from build123d import *

# Parameters (mm, degrees)
CROQUIS1_W              = 100
CROQUIS1_H              = 100
SALIENTE_EXTRUIR1_DEPTH = 10
CROQUIS2_R              = 1.5
CORTAR_EXTRUIR1_DEPTH   = 30
CROQUIS3_W              = 7.071067812
CROQUIS3_H              = 7.071067812
CORTAR_EXTRUIR2_DEPTH   = 8
VACIADO1_START          = -48
VACIADO1_OUTLINE_W      = 8
VACIADO1_OUTLINE_H      = 81.857864376
VACIADO1_DEPTH          = 96
VACIADO1_START_2        = -40.928932188
VACIADO1_2_OUTLINE_W    = 8
VACIADO1_2_OUTLINE_H    = 7.071067812
VACIADO1_2_DEPTH        = 81.857864376


# Read off the part's stored shape, not the designer's step: Vaciado1
with BuildPart() as part:
    # Croquis1 → Saliente-Extruir1 (new body)
    with BuildSketch(Plane(origin=(0, 0, 0), x_dir=(1, 0, 0), z_dir=(0, 1, 0))):
        Rectangle(CROQUIS1_W, CROQUIS1_H)
    extrude(amount=SALIENTE_EXTRUIR1_DEPTH)

    # Croquis2 → Cortar-Extruir1 (cut)
    with BuildSketch(Plane(origin=(0, 10, 0), x_dir=(1, 0, 0), z_dir=(0, 1, 0))):
        with Locations(Location((-46.464466094, -46.464466094, 0), (0, 0, 270))):
            Circle(CROQUIS2_R)
        with Locations(Location((-46.464466094, 46.464466094, 0), (0, 0, 270))):
            Circle(CROQUIS2_R)
        with Locations(Location((46.464466094, 46.464466094, 0), (0, 0, 270))):
            Circle(CROQUIS2_R)
        with Locations(Location((46.464466094, -46.464466094, 0), (0, 0, 270))):
            Circle(CROQUIS2_R)
    extrude(amount=-CORTAR_EXTRUIR1_DEPTH, mode=Mode.SUBTRACT)

    # Croquis3 → Cortar-Extruir2 (cut)
    with BuildSketch(Plane(origin=(0, 10, 0), x_dir=(1, 0, 0), z_dir=(0, 1, 0))):
        with Locations((-46.464466094, -46.464466094)):
            Rectangle(CROQUIS3_W, CROQUIS3_H)
        with Locations((-46.464466094, 46.464466094)):
            Rectangle(CROQUIS3_W, CROQUIS3_H)
        with Locations((46.464466094, 46.464466094)):
            Rectangle(CROQUIS3_W, CROQUIS3_H)
        with Locations((46.464466094, -46.464466094)):
            Rectangle(CROQUIS3_W, CROQUIS3_H)
    extrude(amount=-CORTAR_EXTRUIR2_DEPTH, mode=Mode.SUBTRACT)

    # Vaciado1 outline → Vaciado1 (cut)
    with BuildSketch(Plane.YZ.offset(VACIADO1_START)):
        with Locations((4, 0)):
            Rectangle(VACIADO1_OUTLINE_W, VACIADO1_OUTLINE_H)
    extrude(amount=VACIADO1_DEPTH, mode=Mode.SUBTRACT)

    # Vaciado1 2 outline → Vaciado1 2 (cut)
    with BuildSketch(Plane.YZ.offset(VACIADO1_START_2)):
        with Locations((4, -44.464466094)):
            Rectangle(VACIADO1_2_OUTLINE_W, VACIADO1_2_OUTLINE_H)
        with Locations((4, 44.464466094)):
            Rectangle(VACIADO1_2_OUTLINE_W, VACIADO1_2_OUTLINE_H)
    extrude(amount=VACIADO1_2_DEPTH, mode=Mode.SUBTRACT)


solid = part.part
Part model, mm, in its own coordinate system. A direction names the side the tool comes from. Round coordinates to 2 decimals unless told otherwise and drop trailing zeros. Write each loop counter-clockwise with the first axis right and the second up, starting at its lowest first coordinate (ties: lowest second). Pieces come first, ordered by that corner, then holes. Notation, with made-up numbers: M 85.25,37.25 L 128.25,37.25 A37 ccw 128.25,75.25 Z; hole C 73.25,11.5 d11. An arc over 180 degrees is marked long. Return JSON: item names as keys, results as strings. Group by question number.
(1) Drill centre lines: probe 1 along Z at (x, y) = (41.5, 5.75); probe 2 along X at (y, z) = (7, 11). Where is each one in solid material? Low to high.
(2) Saw through at C-C on z = 37.5. Write the cut outline in (x, y), then the cut area to 3 significant figures.
(3) Saw through at A-A on y = 4. Write the cut outline in (x, z), then the cut area to 3 significant figures.
(4) Saw through at B-B on x = 37. Write the cut outline in (y, z), then the cut area to 3 significant figures.
(5) Pin check, flat tips, straight feed: pin 1 Ø6 at (x, z) = (17, -20) entering from -Y; pin 2 Ø3.5 at (y, z) = (6, 46) entering from +X; pin 3 Ø5.5 at (x, y) = (46.5, 5.5) entering from -Z; pin 4 Ø1.8 at (x, z) = (46.46, 46.46) entering from -Y. Stop position of each tip, or through.
(6) Which spindle directions (+Z, -Z, +X, -X, +Y, -Y) get a long thin tool onto all of the face, cutting with end or side? Do faces 1 (the face through (-48.1, 2, -47.3)), 2 (the face through (-47, 6, 42.929)), 3 (the face through (48, 4, 1)), 4 (the face through (46, 6, -42.929)). Say none if no direction does.
(7) Two-plate mould, pull along X, no slides. Class faces 5 (the face through (42.929, 6, 47)), 6 (the face through (44, 4, 40.929)), 7 (the face through (-50, 5, 1)): +X half, -X half, draft (parallel to the pull), parting line (faces both ways), or undercut.
Returned:
{
 "1": {"probe 1": "-50 to -40.93, 40.93 to 50", "probe 2": "-50 to -48, 48 to 50"},
 "2": {"outline": "M -50,0 L -48,0 L -48,8 L 48,8 L 48,0 L 50,0 L 50,10 L -50,10 Z", "area": "232 mm²"},
 "3": {"outline": "M -50,-42.93 L -42.93,-42.93 L -42.93,-50 L 42.93,-50 L 42.93,-42.93 L 50,-42.93 L 50,42.93 L 42.93,42.93 L 42.93,50 L -42.93,50 L -42.93,42.93 L -50,42.93 Z; hole M -48,-40.93 L -40.93,-40.93 L -40.93,-48 L 40.93,-48 L 40.93,-40.93 L 48,-40.93 L 48,40.93 L 40.93,40.93 L 40.93,48 L -40.93,48 L -40.93,40.93 L -48,40.93 Z", "area": "784 mm²"},
 "4": {"outline": "M 0,-50 L 10,-50 L 10,50 L 0,50 L 0,48 L 8,48 L 8,-48 L 0,-48 Z", "area": "232 mm²"},
 "5": {"pin 1": "y = 8", "pin 2": "x = 42.93", "pin 3": "z = -42.93", "pin 4": "through"},
 "6": {"face 1": "-Z, -X, +Y", "face 2": "+Z, -X, +Y", "face 3": "-Y", "face 4": "-Z, +X, +Y"},
 "7": {"face 5": "+X half", "face 6": "undercut", "face 7": "-X half"}
}
